from build123d import *

# Parameters (mm, degrees)
SKETCH_1_W               = 155
SKETCH_1_H               = 100
EXTRUDE_1_DEPTH          = 5
SKETCH_2_W               = 125
SKETCH_2_H               = 8
EXTRUDE_2_DEPTH          = 25
EXTRUDE_6_DEPTH          = 20
EXTRUDE_7_REACH          = 184.727
EXTRUDE_7_END_RADIUS     = 43.11234224
SKETCH_11_W              = 8
SKETCH_11_H              = 5
SKETCH_12_W              = 125
SKETCH_12_H              = 15
CUT_EXTRUDE_1_DEPTH      = 130
PATTERN_CIRCULAR_1_COUNT = 5
PATTERN_CIRCULAR_1_ANGLE = 90
F_1_THE_OTHER_WAY_COUNT  = 5
F_1_THE_OTHER_WAY_ANGLE  = 90
CUT_EXTRUDE_2_REACH      = 188.145
CUT_EXTRUDE_2_END_RADIUS = 3
SKETCH_17_R              = 0.5
PATTERN_CIRCULAR_2_COUNT = 9
PATTERN_CIRCULAR_2_ANGLE = 180
SKETCH_19_W              = 20
SKETCH_19_H              = 4
CUT_EXTRUDE_3_DEPTH      = 15


with BuildPart() as part:
    # 草图1 → 凸台-拉伸1 (new body)
    with BuildSketch(Plane(origin=(0, 0, 0), x_dir=(1, 0, 0), z_dir=(0, 1, 0))):
        with Locations((77.5, 50)):
            Rectangle(SKETCH_1_W, SKETCH_1_H)
    extrude(amount=EXTRUDE_1_DEPTH)

    # 草图2 → 凸台-拉伸2 (add)
    with BuildSketch(Plane(origin=(0, 5, 0), x_dir=(1, 0, 0), z_dir=(0, 1, 0))):
        with Locations((77.5, 4)):
            Rectangle(SKETCH_2_W, SKETCH_2_H)
    extrude(amount=EXTRUDE_2_DEPTH)

    # 草图7 → 凸台-拉伸6 (add)
    with BuildSketch(Plane(origin=(0, 5, 0), x_dir=(1, 0, 0), z_dir=(0, 1, 0))):
        with BuildLine():
            Line((34.50840207, 68.224369845), (40.49159793, 67.775630155))
            ThreePointArc((40.49159793, 67.775630155), (77.5, 27.88765776), (114.50840207, 67.775630155))
            Line((114.50840207, 67.775630155), (120.49159793, 68.224369845))
            ThreePointArc((120.49159793, 68.224369845), (77.5, 21.88765776), (34.50840207, 68.224369845))
        make_face()
    extrude(amount=EXTRUDE_6_DEPTH)

    # 凸台-拉伸7: up to this cylinder (the profile starts outside it)
    extrude_7_end = Plane(origin=(77.5, 22.5, -65), z_dir=(0, -1, 0)) * Cylinder(EXTRUDE_7_END_RADIUS, 456.67868448, mode=Mode.PRIVATE)
    # 草图11 → 凸台-拉伸7 (add, up to the surface)
    with BuildSketch(Plane(origin=(0, 0, -8), x_dir=(-1, 0, 0), z_dir=(0, 0, -1)), mode=Mode.PRIVATE) as extrude_7_sk1:
        with Locations((-77.5, 22.5)):
            Rectangle(SKETCH_11_W, SKETCH_11_H)
    extrude_7_tool1 = extrude(extrude_7_sk1.sketch, amount=EXTRUDE_7_REACH, mode=Mode.PRIVATE) - extrude_7_end
    add(extrude_7_tool1.solids().sort_by_distance((77.5, 22.5, -8))[0])
    # 草图11 → 凸台-拉伸7 (add, up to the surface)
    with BuildSketch(Plane(origin=(0, 0, -8), x_dir=(-1, 0, 0), z_dir=(0, 0, -1)), mode=Mode.PRIVATE) as extrude_7_sk2:
        with Locations((-41.5, 22.5)):
            Rectangle(SKETCH_11_W, SKETCH_11_H)
    extrude_7_tool2 = extrude(extrude_7_sk2.sketch, amount=EXTRUDE_7_REACH, mode=Mode.PRIVATE) - extrude_7_end
    add(extrude_7_tool2.solids().sort_by_distance((41.5, 22.5, -8))[0])
    # 草图11 → 凸台-拉伸7 (add, up to the surface)
    with BuildSketch(Plane(origin=(0, 0, -8), x_dir=(-1, 0, 0), z_dir=(0, 0, -1)), mode=Mode.PRIVATE) as extrude_7_sk3:
        with Locations((-113.5, 22.5)):
            Rectangle(SKETCH_11_W, SKETCH_11_H)
    extrude_7_tool3 = extrude(extrude_7_sk3.sketch, amount=EXTRUDE_7_REACH, mode=Mode.PRIVATE) - extrude_7_end
    add(extrude_7_tool3.solids().sort_by_distance((113.5, 22.5, -8))[0])

    # 草图12 → 切除-拉伸1 (cut)
    with BuildSketch(Plane(origin=(0, 0, -8), x_dir=(-1, 0, 0), z_dir=(0, 0, -1))):
        with Locations((-77.5, 12.5)):
            Rectangle(SKETCH_12_W, SKETCH_12_H)
    extrude(amount=CUT_EXTRUDE_1_DEPTH, mode=Mode.SUBTRACT)

    # 草图16 → 切除-旋转3 (revolve, cut)
    with BuildSketch(Plane(origin=(0, 18, 0), x_dir=(-1, 0, 0), z_dir=(0, -1, 0))):
        with BuildLine():
            Line((-80.5, 25), (-74.5, 25))
            ThreePointArc((-74.5, 25), (-77.5, 22), (-80.5, 25))
        make_face()
    cut_revolve_3 = revolve(axis=Axis((74.5, 18, -25), (1, 0, 0)), mode=Mode.SUBTRACT)

    # 阵列(圆周)1: 切除-旋转3 ×5 about axis
    pattern_circular_1_axis = Axis((77.5, 0, -65), (0, -1, 0))
    for i in range(1, PATTERN_CIRCULAR_1_COUNT):
        add(cut_revolve_3.rotate(pattern_circular_1_axis, i * PATTERN_CIRCULAR_1_ANGLE / (PATTERN_CIRCULAR_1_COUNT - 1)), mode=Mode.SUBTRACT)

    # 1 the other way: 切除-旋转3 ×5 about axis
    f_1_the_other_way_axis = Axis((77.5, 0, -65), (0, 1, 0))
    for i in range(1, F_1_THE_OTHER_WAY_COUNT):
        add(cut_revolve_3.rotate(f_1_the_other_way_axis, i * F_1_THE_OTHER_WAY_ANGLE / (F_1_THE_OTHER_WAY_COUNT - 1)), mode=Mode.SUBTRACT)

    # 切除-拉伸2: up to this sphere (the profile starts outside it)
    cut_extrude_2_end = Location((37.5, 18, -65)) * Sphere(CUT_EXTRUDE_2_END_RADIUS, mode=Mode.PRIVATE)
    # 草图17 → 切除-拉伸2 (cut, up to the surface)
    with BuildSketch(Plane(origin=(0, 25, 0), x_dir=(1, 0, 0), z_dir=(0, 1, 0)), mode=Mode.PRIVATE) as cut_extrude_2_sk1:
        with Locations(Location((37.5, 64.994842405, 0), (0, 0, 270))):
            Circle(SKETCH_17_R)
    cut_extrude_2_tool1 = extrude(cut_extrude_2_sk1.sketch, amount=-CUT_EXTRUDE_2_REACH, mode=Mode.PRIVATE) - cut_extrude_2_end
    cut_extrude_2 = cut_extrude_2_tool1.solids().sort_by_distance((37.5, 25, -64.994842))[0]
    add(cut_extrude_2, mode=Mode.SUBTRACT)

    # 阵列(圆周)2: 切除-拉伸2 ×9 about axis
    pattern_circular_2_axis = Axis((77.5, 0, -65), (0, 1, 0))
    for i in range(1, PATTERN_CIRCULAR_2_COUNT):
        add(cut_extrude_2.rotate(pattern_circular_2_axis, i * PATTERN_CIRCULAR_2_ANGLE / (PATTERN_CIRCULAR_2_COUNT - 1)), mode=Mode.SUBTRACT)

    # 草图19 → 切除-拉伸3 (cut)
    with BuildSketch(Plane(origin=(0, 30, 0), x_dir=(1, 0, 0), z_dir=(0, 1, 0))):
        with Locations((46.25, 4)):
            Rectangle(SKETCH_19_W, SKETCH_19_H)
        with Locations((108.75, 4)):
            Rectangle(SKETCH_19_W, SKETCH_19_H)
    extrude(amount=-CUT_EXTRUDE_3_DEPTH, mode=Mode.SUBTRACT)


solid = part.part
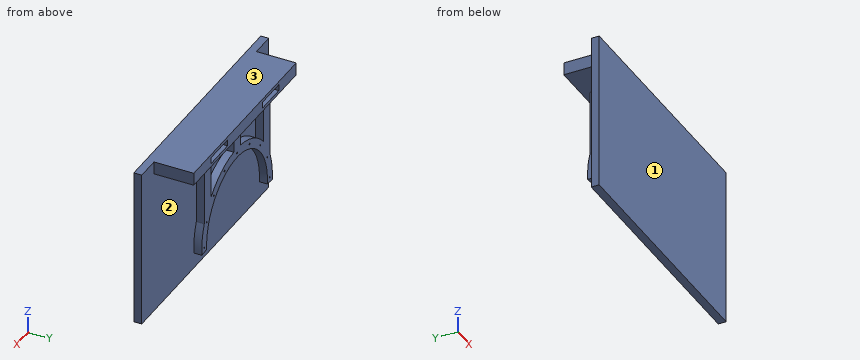
Check sheet for the modelled part. Datum: model origin and axes. Units: mm. Face numbers are marked on the shaded views. Give positions to 0.01 mm unless a question says otherwise; leave off trailing zeros. Loops run counter-clockwise (first coordinate to the right, second up) from the corner with the lowest first, then second, coordinate; pieces in that order, holes last. Notation, with made-up numbers: M 65.25,19.5 L 94.25,19.5 A10 cw 94.25,25.5 Z; hole C 5,7.5 d10. An arc over 180 degrees is marked long. Answer as a JSON object with one key per item and string values. Group by question number.
Q1. Go/stop test with flat-tipped pins: P1, Ø10, axis at x = 95, z = -89.5, coming from the -Y side; P2, Ø1.5, axis at y = 22.5, z = -26, coming from the +X side; P3, Ø4.5, axis at x = 108, y = 20, coming from the -Z side; P4, Ø3, axis at y = 20.5, z = -12.5, coming from the -X side. Record where each tip stops, or that it passes through.
Q2. Material ranges on line 1 along X through (y, z) = (24.75, -64); line 2 along Y through (x, z) = (39.5, -33.5); line 3 along Y through (x, z) = (45, -71.5), recorded low to high. Write a range as [from, to].
Q3. Cross-section at D-D on x = 87. Record the cut outline in (y, z), then the cut area to 3 significant figures.
Q4. Release check for a two-part mould opening along Y. For the marked faces 1, 2 and 3 record: released by +Y, released by -Y, zero draft, split by the parting line, or undercut.
Q5. Cross-section at B-B on y = 27.25. Record the cut outline in (x, z), then the cut area to 3 significant figures.
Q6. Cross-section at A-A on z = -19.5. Record the cut outline in (x, y), then the cut area to 3 significant figures.
Q7. Cross-section at C-C on x = 30.5. Record the cut outline in (y, z).
Evaluation:
{
 "1": {"P1": "stops at y = 0", "P2": "stops at x = 117.5", "P3": "stops at z = -47.54", "P4": "stops at x = 37.5"},
 "2": {"line 1": "x = [34.4, 40.4], [114.6, 120.6]", "line 2": "y = [0, 5], [20, 25]", "line 3": "y = [0, 5]"},
 "3": {"outline": "M 0,-100 L 5,-100 L 5,-8 L 30,-8 L 30,0 L 0,0 Z; M 20,-29.12 L 25,-29.12 L 25,-22.95 L 20,-22.95 Z", "area": "731 mm2"},
 "4": {"face 1": "released by -Y", "face 2": "undercut", "face 3": "zero draft"},
 "5": {"outline": "M 15,-8 L 140,-8 L 140,0 L 15,0 Z; hole M 36.25,-6 L 56.25,-6 L 56.25,-2 L 36.25,-2 Z; hole M 98.75,-6 L 118.75,-6 L 118.75,-2 L 98.75,-2 Z", "area": "840 mm2"},
 "6": {"outline": "M 0,0 L 155,0 L 155,5 L 0,5 Z; M 37.5,20 L 45.5,20 L 45.5,25 L 37.5,25 Z; M 73.5,20 L 81.5,20 L 81.5,25 L 73.5,25 Z; M 109.5,20 L 117.5,20 L 117.5,25 L 109.5,25 Z", "area": "895 mm2"},
 "7": {"outline": "M 0,-100 L 5,-100 L 5,-8 L 30,-8 L 30,0 L 0,0 Z"}
}
